```python
from build123d import *

# Parameters (mm, degrees)
EXTRUDE_THIN1_DEPTH = 555.625
FILLET1_R           = 1.016


with BuildPart() as part:
    # Sketch1 → Extrude-Thin1 (new body)
    with BuildSketch(Plane.XY):
        with BuildLine():
            Line((0, 0), (-3.175, 0))
            ThreePointArc((-3.175, 0), (-4.60251, 2.283581), (-7.14375, 3.175))
            Line((-7.14375, 3.175), (-7.14375, 5.55625))
            ThreePointArc((-7.14375, 5.55625), (-9.525, 7.9375), (-7.14375, 10.31875))
            Line((-7.14375, 10.31875), (-7.14375, 12.7))
            Line((-7.14375, 12.7), (-9.525, 12.7))
            ThreePointArc((-9.525, 12.7), (-11.995981, 23.534537), (-20.091997, 31.146858))
            ThreePointArc((-20.091997, 31.146858), (-23.964886, 34.659641), (-25.4, 39.6875))
            Line((-25.4, 39.6875), (-28.575, 39.6875))
            Line((-28.575, 39.6875), (-28.575, 46.0375))
            Line((-28.575, 46.0375), (-25.4, 46.0375))
            Line((-25.4, 46.0375), (-25.4, 49.2125))
            ThreePointArc((-25.4, 49.2125), (-22.032404, 50.607404), (-20.6375, 53.975))
            Line((-20.6375, 53.975), (-20.6375, 55.5625))
            Line((-20.6375, 55.5625), (-17.4625, 55.5625))
            Line((-17.4625, 55.5625), (-17.4625, 54.5465))
            Line((-17.4625, 54.5465), (-19.6215, 54.5465))
            Line((-19.6215, 54.5465), (-19.6215, 53.975))
            ThreePointArc((-19.6215, 53.975), (-20.969311, 50.265545), (-24.384, 48.28652))
            Line((-24.384, 48.28652), (-24.384, 45.0215))
            Line((-24.384, 45.0215), (-27.559, 45.0215))
            Line((-27.559, 45.0215), (-27.559, 40.7035))
            Line((-27.559, 40.7035), (-24.323126, 40.7035))
            ThreePointArc((-24.323126, 40.7035), (-23.357661, 35.636221), (-19.642184, 32.05786))
            ThreePointArc((-19.642184, 32.05786), (-11.391678, 24.508737), (-8.463037, 13.716))
            Line((-8.463037, 13.716), (-6.12775, 13.716))
            Line((-6.12775, 13.716), (-6.12775, 8.849449))
            ThreePointArc((-6.12775, 8.849449), (-8.509, 7.9375), (-6.12775, 7.025551))
            Line((-6.12775, 7.025551), (-6.12775, 4.088445))
            ThreePointArc((-6.12775, 4.088445), (-3.893771, 3.016555), (-2.431789, 1.016))
            Line((-2.431789, 1.016), (0, 1.016))
            Line((0, 1.016), (0, 0))
        make_face()
    extrude(amount=-EXTRUDE_THIN1_DEPTH)

    # Fillet1
    fillet1_edges = [part.edges().sort_by_distance(p)[0] for p in [
        (-24.323126, 40.7035, -277.8125),
        (-6.12775, 13.716, -277.8125),
        (-6.12775, 8.849449, -277.8125),
        (-6.12775, 7.025551, -277.8125),
        (-3.175, 0, -277.8125),
        (-7.14375, 3.175, -277.8125),
        (-9.525, 12.7, -277.8125),
        (-28.575, 39.6875, -277.8125),
        (-28.575, 46.0375, -277.8125),
        (-25.4, 49.2125, -277.8125),
        (-20.6375, 55.5625, -277.8125),
    ]]
    fillet(fillet1_edges, radius=FILLET1_R)


solid = part.part
```
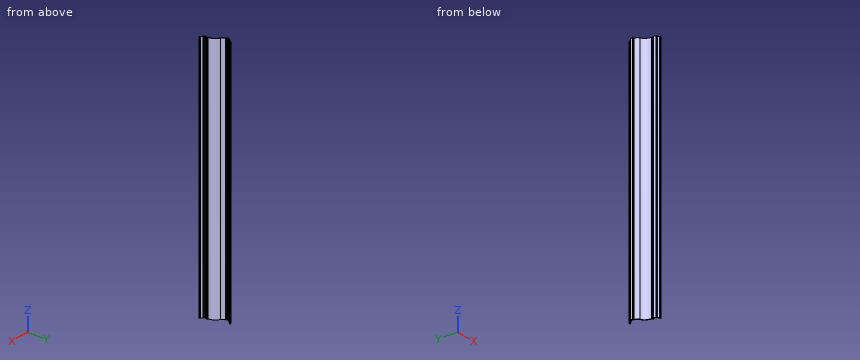
Design review of the part built by this model. Coordinates are the model's own, in mm. Round coordinates to 2 decimals unless told otherwise and drop trailing zeros. Write each loop counter-clockwise with the first axis right and the second up, starting at its lowest first coordinate (ties: lowest second). Pieces come first, ordered by that corner, then holes.
Item 1: For probe 1 along Y at (x, z) = (-25.75, -168); probe 2 along X at (y, z) = (10.5, -153); probe 3 along Y at (x, z) = (-22.5, -377.5), list the stretches that pass through material, from the lowest coordinate up.
Item 2: Clearance check with flat-ended pins moving along their axes: pin 1 Ø0.8 at (y, z) = (55, -241) entering from +X; pin 2 Ø4 at (x, z) = (-17.5, -137) entering from -Y; pin 3 Ø1.6 at (y, z) = (46, -197.5) entering from +X. State where each tip first meets the part, or that it passes through.
Item 3: We need section A-A on y = 19. Write out the cut boundary in (x, z) (3 decimals).
Returned:
1. probe 1: y = 39.69 to 40.7, 45.02 to 46.04
1. probe 2: x = -7.14 to -6.13
1. probe 3: y = 32.84 to 34.35, 48.98 to 50.2
2. pin 1: stops at x = -17.46
2. pin 2: stops at y = 27.97
2. pin 3: stops at x = -24.38
3. outline: (-10.126, -555.625) - (-9.076, -555.625) - (-9.076, 0) - (-10.126, 0) - close
